```python
from build123d import *

# Parameters (mm, degrees)
SKETCH1_R                       = 27
SKETCH1_R_2                     = 9.675
BOSS_EXTRUDE1_DEPTH             = 0.6
SKETCH2_R                       = 9.675
BOSS_EXTRUDE2_DEPTH             = 13.5
SKETCH3_R                       = 10.043523413
SKETCH3_R_2                     = 8
BOSS_EXTRUDE3_DEPTH             = 4.85
CHAMFER1_SIZE                   = 1.5
SKETCH4_R                       = 28.5
SKETCH4_R_2                     = 25
BOSS_EXTRUDE4_DEPTH             = 1.9
BOSS_EXTRUDE4_DIRECTION_2_REACH = 42.704
CHAMFER2_SIZE                   = 1
CHAMFER3_SIZE                   = 1
CUT_EXTRUDE1_DEPTH              = 8.4


with BuildPart() as part:
    # Sketch1 → Boss-Extrude1 (new body)
    with BuildSketch(Plane(origin=(0, 0, 0), x_dir=(1, 0, 0), z_dir=(0, 1, 0))):
        with Locations(Location((0, 0, 0), (0, 0, 270))):
            Circle(SKETCH1_R)
        with Locations(Location((0, 0, 0), (0, 0, 270))):
            Circle(SKETCH1_R_2, mode=Mode.SUBTRACT)
    extrude(amount=BOSS_EXTRUDE1_DEPTH)

    # Sketch2 → Boss-Extrude2 (add)
    with BuildSketch(Plane(origin=(0, 0.6, 0), x_dir=(1, 0, 0), z_dir=(0, 1, 0))):
        Polygon((0, 12.990381057), (-11.25, 6.495190528), (-11.25, -6.495190528), (0, -12.990381057), (11.25, -6.495190528), (11.25, 6.495190528), align=None)
        with Locations(Location((0, 0, 0), (0, 0, 270))):
            Circle(SKETCH2_R, mode=Mode.SUBTRACT)
    extrude(amount=BOSS_EXTRUDE2_DEPTH)

    # Sketch3 → Boss-Extrude3 (add)
    with BuildSketch(Plane(origin=(0, 14.1, 0), x_dir=(1, 0, 0), z_dir=(0, 1, 0))):
        Circle(SKETCH3_R)
        with Locations(Location((0, 0, 0), (0, 0, 270))):
            Circle(SKETCH3_R_2, mode=Mode.SUBTRACT)
    extrude(amount=-BOSS_EXTRUDE3_DEPTH)

    # Chamfer1
    chamfer1_edges = [part.edges().sort_by_distance(p)[0] for p in [
        (0, 9.25, -8),
        (0, 14.1, -8),
        (0, 0, -9.675),
    ]]
    chamfer(chamfer1_edges, length=CHAMFER1_SIZE)

    # Sketch4 → Boss-Extrude4 (add)
    with BuildSketch(Plane.XZ):
        with Locations(Location((0, 0, 0), (0, 0, 270))):
            Circle(SKETCH4_R)
        with Locations(Location((0, 0, 0), (0, 0, 270))):
            Circle(SKETCH4_R_2, mode=Mode.SUBTRACT)
    extrude(amount=BOSS_EXTRUDE4_DEPTH)

    # Boss-Extrude4 direction 2: up to this face of the body (flat: up to its plane)
    boss_extrude4_direction_2_end = Plane(part.part.faces().sort_by_distance((0, 0.6, -26.236324676))[0])
    # Sketch4 → Boss-Extrude4 direction 2 (add, up to the picked face)
    with BuildSketch(Plane.XZ, mode=Mode.PRIVATE) as boss_extrude4_direction_2_sk1:
        with Locations(Location((0, 0, 0), (0, 0, 270))):
            Circle(SKETCH4_R)
        with Locations(Location((0, 0, 0), (0, 0, 270))):
            Circle(SKETCH4_R_2, mode=Mode.SUBTRACT)
    boss_extrude4_direction_2_tool1 = split(extrude(boss_extrude4_direction_2_sk1.sketch, amount=-BOSS_EXTRUDE4_DIRECTION_2_REACH, mode=Mode.PRIVATE), bisect_by=boss_extrude4_direction_2_end, keep=Keep.BOTH, mode=Mode.PRIVATE)
    add(boss_extrude4_direction_2_tool1.solids().sort_by(Axis((0, 0, 27.693898), (0, 1, 0)))[0])

    # Chamfer2
    chamfer2_edges = [part.edges().sort_by_distance(p)[0] for p in [
        (0, 0.6, 28.5),
    ]]
    chamfer(chamfer2_edges, length=CHAMFER2_SIZE)

    # Chamfer3
    chamfer3_edges = [part.edges().sort_by_distance(p)[0] for p in [
        (5.625, 0.6, -9.742785793),
        (-5.625, 0.6, -9.742785793),
        (-11.25, 0.6, 0),
        (-5.625, 0.6, 9.742785793),
        (5.625, 0.6, 9.742785793),
        (11.25, 0.6, 0),
    ]]
    chamfer(chamfer3_edges, length=CHAMFER3_SIZE)

    # Sketch5 → Cut-Extrude1 (cut)
    with BuildSketch(Plane(origin=(0, 0, 0), x_dir=(1, 0, 0), z_dir=(0, 1, 0))):
        with BuildLine():
            ThreePointArc((3.336791258, 24.776315789), (0, 33.5), (-3.336791258, 24.776315789))
            ThreePointArc((-3.336791258, 24.776315789), (0, 25), (3.336791258, 24.776315789))
        make_face()
    extrude(amount=-CUT_EXTRUDE1_DEPTH, mode=Mode.SUBTRACT)


solid = part.part
```
CAD build for the part. Positions are in the model's coordinates, mm. A direction names the side the tool comes from. Coordinates: 2 decimals unless noted, no trailing zeros. Order: outer loops, then holes, each group sorted by start corner. A loop starts at its lowest first (then second) coordinate and runs counter-clockwise, first axis right, second up. Notation, with made-up numbers: M 10,23 L 27,23 A23 ccw 27,60 Z; hole C -33.75,89 d8. An arc over 180 degrees is marked long. Write each question's results on one line, items separated by ' | '. Start each with the question number.
Q1. Cut at C-C (y = 10). List the corners of the cut face in (x, z), then the cut area to 3 significant figures.
Q2. Cut at B-B (y = 6.75). List the corners of the cut face in (x, z) (3 decimals).
Q3. Drill centre lines: probe 1 along X at (y, z) = (6.5, 0) (3 decimals); probe 2 along X at (y, z) = (-1.5, 0); probe 3 along Y at (x, z) = (-21, -6.5). Where is each one in solid material? Low to high. Write a range as from..to.
Q4. Pull direction X, two halves, no side cores. Call faces 4 (the flat face through (-7, 14.1, -7)), 5 (the flat face through (-6, 0, 10)), 6 (the cylindrical face through (0.425, 5.321, -9.666)), 7 (the flat face through (11.25, 8, 0)): +X half, -X half, draft (parallel to the pull), parting line (faces both ways), or undercut.
Q5. Which spindle directions (+Z, -Z, +X, -X, +Y, -Y) get a long thin tool onto all of the face, cutting with end or side? Do faces 1 (the flat face through (-11.25, 8, 0)), 2 (the flat face through (-5.7, 7.8, 9.7)), 3 (the flat face through (13, 0.6, 0)). Say none if no direction does.
Q6. Flat gauge pins, fed straight in: P1, Ø5, axis at y = 4.5, z = 7, coming from the +X side; P2, Ø25, axis at x = 11, z = 11, coming from the -Y side; P3, Ø18.5, axis at x = 0, z = 0, coming from the -Y side; P4, Ø5, axis at y = 0.5, z = 3.5, coming from the -X side. Where does each tip first touch, or does it go through?
Found:
1) outline: M -11.25,-6.5 L 0,-12.99 L 11.25,-6.5 L 11.25,6.5 L 0,12.99 L -11.25,6.5 Z; hole C 0,0 d17.5 | area: 198 mm²
2) outline: M -11.25,-6.495 L 0,-12.99 L 11.25,-6.495 L 11.25,6.495 L 0,12.99 L -11.25,6.495 Z; hole C 0,0 d19.35
3) probe 1: -11.25..-9.675, 9.675..11.25 | probe 2: -28.5..-25, 25..28.5 | probe 3: 0..0.6
4) face 4: draft | face 5: undercut | face 6: undercut | face 7: +X half
5) face 1: +Z, -Z, -X, +Y | face 2: +Z, -X, +Y | face 3: +Y
6) P1: x = 11.25 | P2: y = -1.9 | P3: y = 9.5 | P4: x = -28.48
